Autodesk Inventor part; units mm, degrees
ref_plane "YZ Plane" through (0, 0, 0) normal (1, 0, 0) x (0, 1, 0)
ref_plane "XZ Plane" through (0, 0, 0) normal (0, 1, 0) x (-1, 0, 0)
ref_plane "XY Plane" through (0, 0, 0) normal (0, 0, 1) x (1, 0, 0)
sketch "Sketch1" plane through (0, 0, 0) normal (0, 1, 0) x (-1, 0, 0)
  line L0 (-43.3, -50.05) -> (43.3, -50.05)
  line L1 (43.3, -50.05) -> (43.3, 50.05)
  line L2 (43.3, 50.05) -> (-43.3, 50.05)
  line L3 (-43.3, 50.05) -> (-43.3, -50.05)
  line L4 (-43.3, -50.05) -> (43.3, 50.05) construction
  line L5 (43.3, -50.05) -> (-43.3, 50.05) construction
  point P0 (0, 0)
  dimension "d0" = 86.6
  dimension "d1" = 100.1
extrude "Extrusion1" add sketch "Sketch1" along normal blind 4.445
sketch "Sketch2" plane through (0, 4.445, 0) normal (0, 1, 0) x (1, 0, 0)
  line L0 (40.1, 46.85) -> (-40.1, 46.85)
  line L1 (-40.1, 46.85) -> (-40.1, -46.85)
  line L2 (-40.1, -46.85) -> (40.1, -46.85)
  line L3 (40.1, -46.85) -> (40.1, 46.85)
  line L4 (40.1, 46.85) -> (-40.1, -46.85) construction
  line L5 (-40.1, 46.85) -> (40.1, -46.85) construction
  line L6 (-43.3, 50.05) -> (-43.3, -50.05)
  line L7 (-43.3, -50.05) -> (43.3, -50.05)
  line L8 (43.3, 50.05) -> (-43.3, 50.05)
  line L9 (43.3, -50.05) -> (43.3, 50.05)
  line L10 (36.9, -43.65) -> (43.3, -50.05) construction
  line L11 (34.4431, -46.85) -> (40.4716, -52.8784)
  line L12 (46.1284, -47.2216) -> (40.1, -41.1931)
  arc A0 (40.4716, -52.8784) -> (46.1284, -47.2216) centre (43.3, -50.05) ccw
  circle A1 centre (43.3, -50.05) radius 1.375
  point P0 (0, 0)
  dimension "d4" = 3.2
  dimension "d5" = 3.2
  dimension "d22" = 8
  dimension "d23" = 2.75
extrude "Extrusion2" add sketch "Sketch2" along normal blind 49 contours L0 L1 L2 L11 L7 L6 L8 L9 L12 L3 | L12 L9 A1 L7 L11 L2 L3 | L9 L7 A1 picked at (42.4402, -49.7491)
sketch "Sketch4" plane through (0, 0, 0) normal (0, -1, 0) x (1, 0, 0)
  line L0 (41.7906, 48.7379) -> (44.8094, 51.3621) construction
  line L1 (43.3, 50.05) -> (43.3, -50.05)
  line L2 (43.3, 44.7499) -> (47.4337, 48.3433)
  line L3 (42.1852, 54.381) -> (39.1663, 51.7567)
  arc A0 (39.1663, 51.7567) -> (38.0119, 50.05) centre (41.7906, 48.7379) ccw
  arc A1 (47.4337, 48.3433) -> (42.1852, 54.381) centre (44.8094, 51.3621) ccw
  line L4 (-43.3, 50.05) -> (43.3, 50.05)
  line L5 (38.0119, 50.05) -> (43.3, 50.05)
  line L6 (43.3, 50.05) -> (43.3, 44.7499)
  circle A2 centre (44.8094, 51.3621) radius 1.985
  line L7 (0, 50.05) -> (0, -50.05) construction
  line L8 (43.3, -50.05) -> (-43.3, -50.05) construction
  line L9 (43.3, 0) -> (-33.3, 0) construction
  line L10 (43.3, -50.05) -> (43.3, 50.05)
  line L11 (43.3, -44.7499) -> (47.4337, -48.3433)
  line L12 (42.1852, -54.381) -> (39.1663, -51.7567)
  arc A3 (38.0119, -50.05) -> (39.1663, -51.7567) centre (41.7906, -48.7379) ccw
  arc A4 (42.1852, -54.381) -> (47.4337, -48.3433) centre (44.8094, -51.3621) ccw
  line L13 (-43.3, -50.05) -> (43.3, -50.05)
  circle A5 centre (44.8094, -51.3621) radius 1.985
  line L14 (-43.3, 50.05) -> (-43.3, -50.05)
  line L15 (-43.3, 44.7499) -> (-47.4337, 48.3433)
  line L16 (-42.1852, 54.381) -> (-39.1663, 51.7567)
  arc A6 (-38.0119, 50.05) -> (-39.1663, 51.7567) centre (-41.7906, 48.7379) ccw
  arc A7 (-42.1852, 54.381) -> (-47.4337, 48.3433) centre (-44.8094, 51.3621) ccw
  line L17 (-38.0119, 50.05) -> (-43.3, 50.05)
  circle A8 centre (-44.8094, 51.3621) radius 1.985
  arc A9 (-47.4337, -48.3433) -> (-42.1852, -54.381) centre (-44.8094, -51.3621) ccw
  line L18 (-43.3, -44.7499) -> (-47.4337, -48.3433)
  line L19 (-42.1852, -54.381) -> (-39.1663, -51.7567)
  arc A10 (-39.1663, -51.7567) -> (-38.0119, -50.05) centre (-41.7906, -48.7379) ccw
  circle A11 centre (-44.8094, -51.3621) radius 1.985
  line L20 (-38.0119, -50.05) -> (-43.3, -50.05)
  line L21 (-43.3, -50.05) -> (-43.3, 50.05)
  point P0 (0, 0)
  point P1 (-38.0119, -50.05)
  point P2 (-43.3, -44.7499)
  point P3 (-38.0119, 50.05)
  point P4 (43.3, -44.7499)
  point P5 (43.3, -50.05)
  dimension "d24" = 2
  dimension "d25" = 8
  dimension "d26" = 131
  dimension "d27" = 3.97
extrude "Extrusion4" add sketch "Sketch4" against normal up to surface (53.445 mm away) contours L4 A0 L3 A1 L2 L1 | L11 A4 L12 A3 L13 L1 | L4 L14 L15 A7 L16 A6 | A10 L19 A9 L18 L14 L13
fillet "Fillet2" radius 2 4 edges at (40.1, 28.945, -46.85) (-40.1, 28.945, -46.85) (-40.1, 28.945, 46.85) (40.1, 28.945, 46.85)
sketch "Sketch14" plane through (0, 4.445, 0) normal (0, 1, 0) x (1, 0, 0)
  circle A0 centre (36.6, -34.85) radius 3.7
  circle A1 centre (36.6, -34.85) radius 1.985
  line L0 (38.1, -46.85) -> (-38.1, -46.85)
  line L1 (40.1, 44.85) -> (40.1, -44.85)
  line L2 (-38.1, -46.85) -> (38.1, -46.85) construction
  line L3 (0, -46.85) -> (0, 50.05) construction
  line L4 (38.0119, 50.05) -> (-38.0119, 50.05) construction
  circle A2 centre (36.6, 23.15) radius 3.7
  circle A3 centre (36.6, 23.15) radius 1.985
  line L5 (-40.1, 44.85) -> (-40.1, -44.85) construction
  line L6 (-40.1, 0) -> (40.1, 0) construction
  line L7 (40.1, -44.85) -> (40.1, 44.85) construction
  circle A4 centre (-12.4, -34.85) radius 3.7
  circle A5 centre (-12.4, -34.85) radius 1.985
  circle A6 centre (-12.4, 23.15) radius 1.985
  circle A7 centre (-12.4, 23.15) radius 3.7
  point P0 (0, 0)
  dimension "d114" = 7.4
  dimension "d115" = 3.97
  dimension "d116" = 12
  dimension "d117" = 3.5
  dimension "d120" = 58
  dimension "d127" = 49
sketch "Sketch15" plane through (0, 4.445, 0) normal (0, 1, 0) x (1, 0, 0)
  point P0 (0, 0)
extrude "Extrusion10" add sketch "Sketch14" along normal blind 6
sketch "Sketch16" plane through (43.3, 0, 44.7499) normal (1, 0, 0) x (0, 0, -1)
  line L0 (12.9515, 13.2621) -> (12.9515, 13.455)
  line L1 (20.9323, 13.455) -> (20.9323, 13.2621)
  line L2 (13.9419, 14.5004) -> (19.9419, 14.5004)
  line L3 (88.3241, 11.975) -> (9.3999, 11.975)
  line L4 (22.9323, 9.975) -> (10.9515, 9.975)
  line L5 (10.9515, 9.975) -> (10.9515, 19.0004)
  line L6 (10.9515, 19.0004) -> (22.9323, 19.0004)
  line L7 (22.9323, 19.0004) -> (22.9323, 9.975)
  line L8 (30.8419, 17.055) -> (30.8419, 14.5766)
  line L9 (45.8419, 14.5766) -> (45.8419, 17.055)
  line L10 (45.0419, 17.855) -> (31.6419, 17.855)
  line L11 (47.8419, 10.975) -> (28.8419, 10.975)
  line L12 (28.8419, 10.975) -> (28.8419, 19.855)
  line L13 (28.8419, 19.855) -> (47.8419, 19.855)
  line L14 (47.8419, 19.855) -> (47.8419, 10.975)
  line L15 (56.4419, 17.775) -> (56.4419, 11.775)
  line L16 (63.4419, 11.775) -> (63.4419, 17.775)
  line L17 (63.4419, 17.775) -> (59.9419, 17.775)
  line L18 (59.9419, 17.775) -> (56.4419, 17.775)
  line L19 (64.9419, 10.975) -> (54.9419, 10.975)
  line L20 (54.9419, 10.975) -> (54.9419, 19.275)
  line L21 (54.9419, 19.275) -> (64.9419, 19.275)
  line L22 (64.9419, 19.275) -> (64.9419, 10.975)
  point P0 (44.7499, 0)
  dimension "d134" = 4.5
  dimension "d135" = 2
  dimension "d136" = 2
  dimension "d137" = 2
  dimension "d138" = 2
  dimension "d139" = 1
  dimension "d140" = 2
  dimension "d141" = 2
  dimension "d142" = 1
  dimension "d143" = 1.5
  dimension "d144" = 1.5
  dimension "d145" = 1.5
extrude "Extrusion11" cut sketch "Sketch16" against normal up to surface (3.2 mm away)
sketch "Sketch17" plane through (38.0119, 0, -50.05) normal (0, 0, -1) x (-1, 0, 0)
  line L0 (16.1912, 11.975) -> (16.1912, 25.475)
  line L1 (0.3112, 11.975) -> (0.3112, 25.475)
  line L2 (0.3112, 25.475) -> (16.1912, 25.475)
  line L3 (50.9119, 11.975) -> (0.9119, 11.975)
  line L4 (16.4912, 11.725) -> (0.0112, 11.725)
  line L5 (0.0112, 11.725) -> (0.0112, 25.725)
  line L6 (0.0112, 25.725) -> (16.4912, 25.725)
  line L7 (16.4912, 25.725) -> (16.4912, 11.725)
  line L8 (19.4512, 18.7546) -> (19.4512, 21.7546)
  line L9 (34.5512, 21.7546) -> (34.5512, 18.7546)
  line L10 (24.0012, 27.465) -> (30.0012, 27.465)
  line L11 (35.2512, 11.225) -> (18.7512, 11.225)
  line L12 (18.7512, 11.225) -> (18.7512, 28.465)
  line L13 (18.7512, 28.465) -> (35.2512, 28.465)
  line L14 (35.2512, 28.465) -> (35.2512, 11.225)
  line L15 (37.4512, 18.7546) -> (37.4512, 21.7546)
  line L16 (52.5512, 21.7546) -> (52.5512, 18.7546)
  line L17 (42.0012, 27.465) -> (48.0012, 27.465)
  line L18 (53.2512, 11.225) -> (36.7512, 11.225)
  line L19 (36.7512, 11.225) -> (36.7512, 28.465)
  line L20 (36.7512, 28.465) -> (53.2512, 28.465)
  line L21 (53.2512, 28.465) -> (53.2512, 11.225)
  point P0 (38.0119, 0)
  point P1 (18.7512, 11.975)
  point P2 (35.2512, 11.975)
  dimension "d148" = 0.3
  dimension "d149" = 0.3
  dimension "d150" = 0.25
  dimension "d151" = 0.25
  dimension "d154" = 0.7
  dimension "d155" = 0.7
  dimension "d156" = 1
  dimension "d157" = 0.75
  dimension "d158" = 1
  dimension "d159" = 0.7
  dimension "d160" = 0.7
  dimension "d161" = 0.75
extrude "Extrusion12" cut sketch "Sketch17" against normal up to surface (3.2 mm away)
sketch "Sketch19" plane through (-43.3, 0, -44.7499) normal (-1, 0, 0) x (0, 0, 1)
  circle A0 centre (20, 25) radius 9.6
  line L0 (0, 53.445) -> (0, 0)
  line L1 (0, 0) -> (89.4999, 0)
  point P0 (44.7499, 0)
  dimension "d162" = 19.2
  dimension "d163" = 20
  dimension "d164" = 25
extrude "Extrusion13" cut sketch "Sketch19" against normal up to surface (3.2 mm away)
sketch "Sketch20" plane through (-43.3, 0, -44.7499) normal (-1, 0, 0) x (0, 0, 1)
  line L0 (0, 53.445) -> (89.4999, 53.445)
  line L1 (81.3249, 15.625) -> (54.2749, 15.625)
  line L2 (54.2749, 15.625) -> (54.2749, 34.375)
  line L3 (54.2749, 34.375) -> (81.3249, 34.375)
  line L4 (81.3249, 34.375) -> (81.3249, 15.625)
  line L5 (81.3249, 15.625) -> (54.2749, 34.375) construction
  line L6 (54.2749, 15.625) -> (81.3249, 34.375) construction
  line L7 (81.4999, 11.15) -> (54.0999, 11.15)
  line L8 (54.0999, 11.15) -> (54.0999, 38.85)
  line L9 (54.0999, 38.85) -> (81.4999, 38.85)
  line L10 (81.4999, 38.85) -> (81.4999, 11.15)
  line L11 (81.4999, 11.15) -> (54.0999, 38.85) construction
  line L12 (54.0999, 11.15) -> (81.4999, 38.85) construction
  line L13 (0, 0) -> (89.4999, 0)
  line L14 (89.4999, 0) -> (89.4999, 53.445)
  circle A0 centre (56.0999, 36.85) radius 1
  line L15 (67.7999, 34.375) -> (67.7999, 11.15) construction
  line L16 (54.0999, 25) -> (81.4999, 25) construction
  circle A1 centre (79.4999, 36.85) radius 1
  circle A2 centre (56.0999, 13.15) radius 1
  circle A3 centre (79.4999, 13.15) radius 1
  point P0 (44.7499, 0)
  point P1 (67.7999, 25)
  dimension "d195" = 27.05
  dimension "d196" = 18.75
  dimension "d197" = 27.7
  dimension "d198" = 27.4
  dimension "d199" = 25
  dimension "d200" = 8
  dimension "d203" = 2
  dimension "d204" = 2
  dimension "d205" = 2
extrude "Extrusion16" cut sketch "Sketch20" against normal up to surface (3.2 mm away) contours L1 L2 L3 L4 | A0 | A1 | A2 | A3
properties part number "_3DPrint"
The listing builds one solid part. Answer for the finished solid, in the listing's coordinates (mm). A direction names the side the tool comes from. Coordinates: 2 decimals unless noted, no trailing zeros. Order: outer loops, then holes, each group sorted by start corner. A loop starts at its lowest first (then second) coordinate and runs counter-clockwise, first axis right, second up.
Q1. A cutting plane is placed at D-D, the plane y = 49. State how many separate pieces and enclosed holes the cut face has, and give its area (3 significant figures).
Q2. A cutting plane is placed at A-A, the plane x = 15. Write down the section's boundary in (y, z) (3 decimals), and give its area (3 significant figures).
Q3. Which of the six approach directions +Z, -Z, +X, -X, +Y, -Y give full straight-line access (tool end or side, diameter ignored) to faces 1 (the face through (-42, 25, 9.525)), 2 (the face through (-1, 26, 50.05)), 3 (the face through (40.7, 26.35, -53.09)), 4 (the face through (-15.239, 20, -48)), 5 (the face through (38.05, 10.445, 36.44))?
Q4. Given P1, Ø12, axis at y = 44, z = -40.5, coming from the +X side; P2, Ø2, axis at x = -14.5, z = 4, coming from the +Y side (3 decimals); P3, Ø16, axis at y = 36, z = 4, coming from the +X side; P4, Ø2.5, axis at x = -44.81, z = -51.36, coming from the -Y side, each flat-ended and moving along its own axis, determine where each tip first touches the part or whether it passes through.
Q5. For a pull along Y with two mould halves and no side action, classify faces 6 (the face through (40.7, 26.35, 53.09)), 7 (the face through (30, 11.725, -48)), 8 (the face through (-12, 4.445, 35)) as pulls with the +Y half, pulls with the -Y half, needs draft (parallel to the pull), parting line crosses it, or undercut.
Q6. Consider line 1 (X direction, y = 9.25, z = -23.15) (3 decimals); line 2 (Y direction, x = -41.55, z = 34.75) (3 decimals); line 3 (X direction, y = 19, z = 38). Determine where each line is inside the solid, lowest interval first.
Q7. A cutting plane is placed at B-B, the plane z = 20. Write down the section's boundary in (x, y) (3 decimals), and give its area (3 significant figures).
Q8. A cutting plane is placed at C-C, the plane x = -23. Write down the section's boundary in (y, z) (3 decimals).
Answers follow:
1. separate pieces: 1
1. enclosed holes: 5
1. area: 1,330 mm2
2. outline: (0, -50.05) - (11.225, -50.05) - (11.225, -46.85) - (4.445, -46.85) - (4.445, 46.85) - (53.445, 46.85) - (53.445, 50.05) - (0, 50.05) - close; (28.465, -50.05) - (53.445, -50.05) - (53.445, -46.85) - (28.465, -46.85) - close
2. area: 703 mm2
3. face 1: -X
3. face 2: +Z, +Y, -Y
3. face 3: -Z, +Y, -Y
3. face 4: -Z
3. face 5: +Y
4. P1: stops at x = 45.31
4. P2: stops at y = 4.445
4. P3: stops at x = 43.3
4. P4: passes through
5. face 6: needs draft
5. face 7: undercut
5. face 8: pulls with the +Y half
6. line 1: x = -43.3 to -40.1, -16.1 to -14.385, -10.415 to -8.7, 32.9 to 34.615, 38.585 to 43.3
6. line 2: y = 0 to 12.15, 14.15 to 15.625, 34.375 to 35.85, 37.85 to 53.445
6. line 3: x = -43.3 to -40.1, 40.1 to 43.3
7. outline: (-43.3, 0) - (43.3, 0) - (43.3, 53.445) - (40.1, 53.445) - (40.1, 4.445) - (-40.1, 4.445) - (-40.1, 15.625) - (-43.3, 15.625) - close; (-43.3, 34.375) - (-40.1, 34.375) - (-40.1, 53.445) - (-43.3, 53.445) - close
7. area: 639 mm2
8. outline: (0, -50.05) - (53.445, -50.05) - (53.445, -46.85) - (4.445, -46.85) - (4.445, 46.85) - (53.445, 46.85) - (53.445, 50.05) - (0, 50.05) - close
